For this review, take the finished solid that the model builds, in its own axes (mm). A direction names the side the tool comes from. Round coordinates to 2 decimals unless told otherwise and drop trailing zeros. Loops run counter-clockwise (first coordinate to the right, second up) from the corner with the lowest first, then second, coordinate; pieces in that order, holes last. Notation, with made-up numbers: (6.25, -16) -> (29.25, -16) arc R7 cw to (29.25, -3) -> close; hole circle Ø8 at (42, 46.25). An arc over 180 degrees is marked (long way). Use one line per item in the form item = value. Start each with the question number.
from build123d import *

# Parameters (mm, degrees)
CONG_1_R           = 1.5
CONG_2_R           = 3
COQUE1_START       = 10.264335876
COQUE1_2_OUTLINE_R = 6
COQUE1_2_DEPTH     = 1.041752411
COQUE1_3_OUTLINE_R = 6
COQUE1_3_DEPTH     = 10.264335876
COQUE1_START_2     = 11.306088287
COQUE1_4_OUTLINE_R = 6
COQUE1_4_DEPTH     = 2.140756903


with BuildPart() as part:
    # Esquisse1 → R_volution1 (revolve)
    with BuildSketch(Plane.XY, mode=Mode.PRIVATE) as r_volution1_sk:
        Polygon((10, 0), (10, 7.060491131), (11.528559936, 12.44684519), (5, 12.44684519), (5, 0), align=None)
    revolve(r_volution1_sk.sketch.rotate(Axis((5, 0, 0), (0, 1, 0)), 90), axis=Axis((5, 0, 0), (0, 1, 0)))

    # Cong_1
    cong_1_edges = [part.edges().sort_by_distance(p)[0] for p in [
        (5, 12.44684519, 6.528559936),
    ]]
    fillet(cong_1_edges, radius=CONG_1_R)

    # Cong_2
    cong_2_edges = [part.edges().sort_by_distance(p)[0] for p in [
        (5, 7.060491131, 5),
    ]]
    fillet(cong_2_edges, radius=CONG_2_R)

    # Coque1: read off the stored shape, not the designer's step
    # Coque1 outline → Coque1 (revolve)
    with BuildSketch(Plane(origin=(5, 0, 0), x_dir=(1, 0, 0), z_dir=(0, 0, 1))):
        with BuildLine():
            Line((6, 12.978852966), (6, 6.643057066))
            ThreePointArc((6, 6.643057066), (6.019084561, 6.918690928), (6.075974025, 7.189064438))
            Line((6.075974025, 7.189064438), (6.948686219, 10.264335976))
            ThreePointArc((6.948686219, 10.264335976), (6.903677484, 11.771640909), (6, 12.978852966))
        make_face()
    revolve(axis=Axis((5, 0, 0), (0, 1, 0)))

    # Coque1 2 outline → Coque1 2 (cut)
    with BuildSketch(Plane(origin=(0, 0, 0), x_dir=(1, 0, 0), z_dir=(0, 1, 0)).offset(COQUE1_START)):
        with Locations((5, 0)):
            Circle(COQUE1_2_OUTLINE_R)
    extrude(amount=COQUE1_2_DEPTH, mode=Mode.SUBTRACT)

    # Coque1 3 outline → Coque1 3 (add)
    with BuildSketch(Plane(origin=(0, 0, 0), x_dir=(1, 0, 0), z_dir=(0, 1, 0))):
        with Locations((5, 0)):
            Circle(COQUE1_3_OUTLINE_R)
    extrude(amount=COQUE1_3_DEPTH)

    # Coque1 4 outline → Coque1 4 (add)
    with BuildSketch(Plane(origin=(0, 0, 0), x_dir=(1, 0, 0), z_dir=(0, 1, 0)).offset(COQUE1_START_2)):
        with Locations((5, 0)):
            Circle(COQUE1_4_OUTLINE_R)
    extrude(amount=COQUE1_4_DEPTH)

    # Coque1 5 outline → Coque1 5 (revolve, cut)
    with BuildSketch(Plane(origin=(5, 0, 0), x_dir=(1, 0, 0), z_dir=(0, 0, 1))):
        with BuildLine():
            Line((6, 11.306088287), (6, 10.587602092))
            ThreePointArc((6, 10.587602092), (6.043653751, 10.94684519), (6, 11.306088287))
        make_face()
        with BuildLine():
            Line((5.113961038, 7.462068123), (5.909199194, 10.264335909))
            Line((5.909199194, 10.264335909), (0, 10.264335909))
            Line((0, 10.264335909), (0, 0))
            Line((0, 0), (5, 0))
            Line((5, 0), (5, 6.643057066))
            ThreePointArc((5, 6.643057066), (5.028626842, 7.056507858), (5.113961038, 7.462068123))
        make_face()
        with BuildLine():
            ThreePointArc((6, 11.306088287), (5.468622765, 12.12770603), (4.543653751, 12.44684519))
            Line((4.543653751, 12.44684519), (0, 12.44684519))
            Line((0, 12.44684519), (0, 11.306088287))
            Line((0, 11.306088287), (6, 11.306088287))
        make_face()
        with BuildLine():
            Line((6, 12.978852966), (6, 13.44684519))
            Line((6, 13.44684519), (4.543653751, 13.44684519))
            ThreePointArc((4.543653751, 13.44684519), (5.308500324, 13.326973279), (6, 12.978852966))
        make_face()
    revolve(axis=Axis((5, 0, 0), (0, 1, 0)), mode=Mode.SUBTRACT)

    # Coque1 6 outline → Coque1 6 (revolve)
    with BuildSketch(Plane(origin=(5, 0, 0), x_dir=(1, 0, 0), z_dir=(0, 0, 1))):
        with BuildLine():
            Line((5.909199194, 10.264335876), (6, 10.264335876))
            Line((6, 10.264335876), (6, 10.587602092))
            ThreePointArc((6, 10.587602092), (5.993554433, 10.562413124), (5.986673232, 10.537339662))
            Line((5.986673232, 10.537339662), (5.909199194, 10.264335876))
        make_face()
    revolve(axis=Axis((5, 0, 0), (0, 1, 0)))


solid = part.part
Item 1: Wall thickness on line 1 (Z direction, x = 5, y = 2.25); line 2 (X direction, y = 1.5, z = 0); line 3 (Y direction, x = 4.75, z = -2): over which ranges is each line inside the solid? List them lowest first.
Item 2: Take a section at B-B on y = 12.25. Give the boundary of the cut face in (x, z).
Item 3: Take a section at A-A on y = 1.75. Give the boundary of the cut face in (x, z), plus the area to 3 significant figures.
Item 4: Machinability: for faces 4 (the flat face through (5, 12.447, 0)), 5 (the flat face through (1, 0, -4)), which of the approach directions +Z, -Z, +X, -X, +Y, -Y give a long, thin tool a straight path to every point of the face, cutting with its end or side? Answer none if there is none.
Item 5: For P1, Ø5, axis at x = 8, y = 11, coming from the -Z side; P2, Ø8, axis at y = 12, z = -4, coming from the -X side; P3, Ø2, axis at y = 10.5, z = 4.5, coming from the +X side; P4, Ø1, axis at x = 3, z = 5, coming from the -Y side, all flat-tipped, find the tip position at first contact; note any pin that passes through.
Item 6: Draft analysis for pull direction X (two halves, no side actions). For faces 1 (the cylindrical face through (-1, 3, 0)), 2 (the cylindrical face through (0, 3, 0)), 3 (the flat face through (5, 13.447, 0)), state which applies: +X half, -X half, draft (parallel to the pull), parting line (faces both ways), or undercut.
Results:
q1.line_1 = -6 to -5, 5 to 6
q1.line_2 = -1 to 0, 10 to 11
q1.line_3 = 12.45 to 13.45
q2.outline = circle Ø13.35 at (5, 0); hole circle Ø10.57 at (5, 0)
q3.outline = circle Ø12 at (5, 0); hole circle Ø10 at (5, 0)
q3.area = 34.6 mm2
q4.face_4 = -Y
q4.face_5 = +Z, -Z, +X, -X, -Y
q5.P1 = -7.03
q5.P2 = -2.04
q5.P3 = 11.09
q5.P4 = 0
q6.face_1 = parting line
q6.face_2 = undercut
q6.face_3 = draft
